from build123d import *

# Parameters (mm, degrees)
F1_DEPTH = 640
F3_DEPTH = 258
F5_DEPTH = 1440


with BuildPart() as f1:
    # F0 (on Front) → F1 (new body)
    with BuildSketch(Plane.XZ):
        Polygon((-576.332047, -28.611164), (-565.888931, -378.455331), (594.111069, -378.455331), (594.111069, -32.202492), (192.212863, 262.286696), align=None)
    extrude(amount=F1_DEPTH)

    # F2 (on face) → F3 (join)
    with BuildSketch(Plane(origin=(0, 0, 0), x_dir=(-1, 0, 0), z_dir=(0, 1, 0))):
        Polygon((223.529473, -133.722216), (-594.111069, -32.202492), (-594.111069, -378.455331), (223.529473, -378.455331), align=None)
    extrude(amount=F3_DEPTH)

    # F4 (on face) → F5 (cut)
    with BuildSketch(Plane(origin=(-576.672258, 0, -17.214108), x_dir=(0, -1, 0), z_dir=(-0.999555, 0, -0.029837))):
        with BuildLine():
            Line((128.456429, -201.147199), (130.758941, -361.402132))
            Line((130.758941, -361.402132), (517.019868, -361.402132))
            Line((517.019868, -361.402132), (517.019868, -201.147199))
            ThreePointArc((517.019868, -201.147199), (322.738148, -95.409288), (128.456429, -201.147199))
        make_face()
    extrude(amount=-F5_DEPTH, mode=Mode.SUBTRACT)


solid = f1.part
Work out the finished part from the listing and answer in its coordinate system (mm). A direction names the side the tool comes from. Round coordinates to 2 decimals unless told otherwise and drop trailing zeros. Write each loop counter-clockwise with the first axis right and the second up, starting at its lowest first coordinate (ties: lowest second). Pieces come first, ordered by that corner, then holes. Notation, with made-up numbers: M 43.5,65.5 L 100.5,65.5 A24 ccw 100.5,78.5 Z; hole C -15.75,-32 d9. An arc over 180 degrees is marked long. Use a Markdown table: item, result.
1) Determine the mould class of faces 5 (the face through (6, -517.02, -282)), 6 (the face through (1, -640, -125)), 7 (the face through (395.975, -315.52, 112.981)) for opening direction Z: pulls with the +Z half, pulls with the -Z half, needs draft (parallel to the pull), parting line crosses it, or undercut.
Taken from the geometry:
| item | result |
|---|---|
| face 5 | undercut |
| face 6 | needs draft |
| face 7 | pulls with the +Z half |
2) Consider line 1 (Y direction, x = -72.5, z = 156); line 2 (Z direction, x = -112, y = -206); line 3 (X direction, y = 139.5, z = -147). Determine where each line is inside the solid, lowest interval first. Write a range as [from, to].
Taken from the geometry:
| item | result |
|---|---|
| line 1 | y = [-640, 0] |
| line 2 | z = [-378.46, -364.91], [-130.42, 147.14] |
| line 3 | x = [-223.53, 594.11] |
3) Flat-ended cylindrical pins translate along their axes: pin 1 (10 mm diameter, centred on x = 287, y = -150.5, fed in from +Z); pin 2 (2 mm diameter, centred on x = -365, z = 49, fed in from +Y); pin 3 (2 mm diameter, centred on x = -18, y = 4.5, fed in from +Z). Find the tip coordinate at first contact, or state that the pin passes through.
Taken from the geometry:
| item | result |
|---|---|
| pin 1 | stops at z = 196.5 |
| pin 2 | stops at y = 0 |
| pin 3 | stops at z = -108.08 |
4) Which of the six approach directions +Z, -Z, +X, -X, +Y, -Y give full straight-line access (tool end or side, diameter ignored) to faces 1 (the face through (2.22, -325.97, -95.41)), 2 (the face through (-223.529, 127, -258)), 3 (the face through (179.567, 127.194, -83.673)), 4 (the face through (-186.68, -315.52, 118.874))?
Taken from the geometry:
| item | result |
|---|---|
| face 1 | +X |
| face 2 | +Z, -Z, -X, +Y |
| face 3 | +Z, -X, +Y |
| face 4 | +Z, -X, +Y, -Y |
5) The part is cut by section B-B on y = -89.5. Give the vertices of the cut face in (x, z), plus the area to 3 significant figures.
Taken from the geometry:
| item | result |
|---|---|
| outline | M -576.33,-28.61 L -565.89,-378.46 L 594.11,-378.46 L 594.11,-32.2 L 192.21,262.29 Z |
| area | 577,000 mm2 |
6) The part is cut by section C-C on z = -58. Give the vertices of the cut face in (x, y).
Taken from the geometry:
| item | result |
|---|---|
| outline | M -575.45,-640 L 594.11,-640 L 594.11,258 L 386.34,258 L 386.34,0 L -575.45,0 Z |
7) The part is cut by section A-A on y = -490. Give the vertices of the cut face in (x, z), plus the area to 3 significant figures.
Taken from the geometry:
| item | result |
|---|---|
| outline | M -576.33,-28.61 L -571.69,-184.06 L 594.11,-149.27 L 594.11,-32.2 L 192.21,262.29 Z; M -565.89,-378.46 L 594.11,-378.46 L 594.11,-343.83 Z |
| area | 351,000 mm2 |
8) The part is cut by section D-D on y = -281. Give the vertices of the cut face in (x, z), plus the area to 3 significant figures.
Taken from the geometry:
| item | result |
|---|---|
| outline | M -576.33,-28.61 L -573.71,-116.38 L 594.11,-81.52 L 594.11,-32.2 L 192.21,262.29 Z; M -565.89,-378.46 L 594.11,-378.46 L 594.11,-343.83 Z |
| area | 272,000 mm2 |
